The model under review builds one solid part; all positions refer to its coordinate system, in mm. Face numbers are marked on the shaded views. A direction names the side the tool comes from. Coordinates: 2 decimals unless noted, no trailing zeros. Loops run counter-clockwise (first coordinate to the right, second up) from the corner with the lowest first, then second, coordinate; pieces in that order, holes last. Notation, with made-up numbers: M 24.25,59 L 32.25,59 A28 ccw 32.25,80 Z; hole C 16,-11 d6. An arc over 180 degrees is marked long. Return JSON: item names as keys, results as strings.
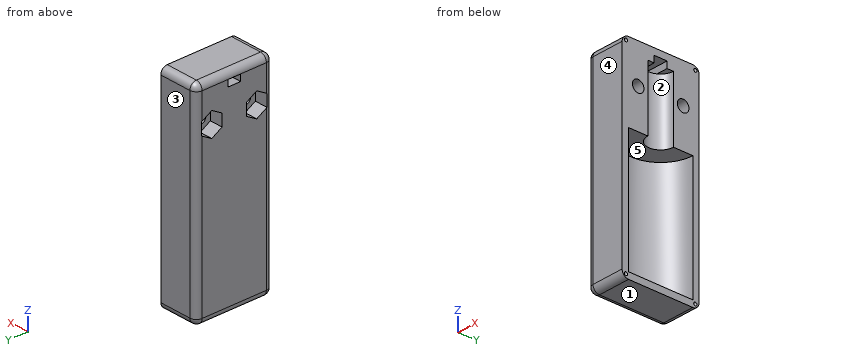
```python
from build123d import *

# Parameters (mm, degrees)
SKETCH1_W               = 6
SKETCH1_H               = 12
BOSS_EXTRUDE1_DEPTH     = 20
SKETCH2_R               = 5
CUT_EXTRUDE1_DEPTH      = 19
SKETCH6_W               = 6
SKETCH6_H               = 12
BOSS_EXTRUDE3_DEPTH     = 12
SKETCH7_R               = 2
CUT_EXTRUDE2_DEPTH      = 10
CUT_EXTRUDE3_DEPTH      = 25.083189158
CUT_EXTRUDE3_DEPTH_BACK = 25.083189158
SKETCH8_W               = 1
SKETCH8_H               = 2
FILLET1_R               = 1
SKETCH10_R              = 0.9
CUT_EXTRUDE4_DEPTH      = 10
CUT_EXTRUDE5_DEPTH      = 2


with BuildPart() as part:
    # Sketch1 → Boss-Extrude1 (new body)
    with BuildSketch(Plane.XY):
        with Locations((3, 6)):
            Rectangle(SKETCH1_W, SKETCH1_H)
    extrude(amount=-BOSS_EXTRUDE1_DEPTH)

    # Sketch2 → Cut-Extrude1 (cut)
    with BuildSketch(Plane.XY):
        with Locations((6, 6)):
            Circle(SKETCH2_R)
    extrude(amount=-CUT_EXTRUDE1_DEPTH, mode=Mode.SUBTRACT)

    # Sketch6 → Boss-Extrude3 (add)
    with BuildSketch(Plane.XY):
        with Locations((3, 6)):
            Rectangle(SKETCH6_W, SKETCH6_H)
    extrude(amount=BOSS_EXTRUDE3_DEPTH)

    # Sketch7 → Cut-Extrude2 (cut)
    with BuildSketch(Plane(origin=(0, 0, 0), x_dir=(-1, 0, 0), z_dir=(0, 0, -1))):
        with Locations((-6, 6)):
            Circle(SKETCH7_R)
    extrude(amount=-CUT_EXTRUDE2_DEPTH, mode=Mode.SUBTRACT)

    # Sketch8 → Cut-Extrude3 (cut, two sides: drawn at the far end of the back side and taken through both)
    with BuildSketch(Plane.ZY.offset(-CUT_EXTRUDE3_DEPTH_BACK)):
        with Locations((10.5, 6)):
            Rectangle(SKETCH8_W, SKETCH8_H)
    extrude(amount=CUT_EXTRUDE3_DEPTH + CUT_EXTRUDE3_DEPTH_BACK, mode=Mode.SUBTRACT)

    # Fillet1
    fillet1_edges = [part.edges().sort_by_distance(p)[0] for p in [
        (3, 0, -20),
        (3, 12, 12),
        (0, 6, 12),
        (3, 0, 12),
        (0, 6, -20),
        (0, 0, -4),
        (0, 12, -4),
        (3, 12, -20),
    ]]
    fillet(fillet1_edges, radius=FILLET1_R - 0.0001)  # a hair under: the kernel refuses the full size

    # Sketch10 → Cut-Extrude4 (cut)
    with BuildSketch(Plane(origin=(6, 0, 0), x_dir=(0, 0, -1), z_dir=(1, 0, 0))):
        with Locations((-6, 9.5)):
            Circle(SKETCH10_R)
    cut_extrude4 = extrude(amount=-CUT_EXTRUDE4_DEPTH, mode=Mode.SUBTRACT)

    # Sketch12 → Cut-Extrude5 (cut)
    with BuildSketch(Plane.ZY):
        Polygon((6.923760431, 7.9), (7.847520861, 9.5), (6.923760431, 11.1), (5.076239569, 11.1), (4.152479139, 9.5), (5.076239569, 7.9), align=None)
    cut_extrude5 = extrude(amount=-CUT_EXTRUDE5_DEPTH, mode=Mode.SUBTRACT)

    # Mirror1: Cut-Extrude4, Cut-Extrude5 across plane
    add(cut_extrude4.mirror(Plane.ZX.offset(6)), mode=Mode.SUBTRACT)
    add(cut_extrude5.mirror(Plane.ZX.offset(6)), mode=Mode.SUBTRACT)

    # Sketch11 → Cut-Revolve1 (revolve, cut)
    with BuildSketch(Plane(origin=(0, 0, -19.4), x_dir=(-1, 0, 0), z_dir=(0, 0, -1))):
        with BuildLine():
            Line((-5.75, 11.4), (-6, 11.4))
            Line((-6, 11.4), (-6, 11.15))
            ThreePointArc((-6, 11.15), (-5.823223305, 11.223223305), (-5.75, 11.4))
        make_face()
    cut_revolve1 = revolve(axis=Axis((5.75, 11.4, -19.4), (1, 0, 0)), mode=Mode.SUBTRACT)

    # Mirror2: Cut-Revolve1 across plane
    add(cut_revolve1.mirror(Plane.ZX.offset(6)), mode=Mode.SUBTRACT)

    # Mirror2 at the second plane: Cut-Revolve1 across plane
    add(cut_revolve1.mirror(Plane.XY.offset(-4)), mode=Mode.SUBTRACT)

    # Mirror2 at the second plane copy 1 sketc → Mirror2 at the second plane copy 1 (revolve, cut)
    with BuildSketch(Plane(origin=(0, 12, 11.4), x_dir=(-1, 0, 0), z_dir=(0, 0, 1))):
        with BuildLine():
            Line((-5.75, 11.4), (-6, 11.4))
            Line((-6, 11.4), (-6, 11.15))
            ThreePointArc((-6, 11.15), (-5.823223305, 11.223223305), (-5.75, 11.4))
        make_face()
    revolve(axis=Axis((5.75, 0.6, 11.4), (1, 0, 0)), mode=Mode.SUBTRACT)


solid = part.part
```
1. Add section B-B on z = 6. Give the boundary of the cut face in (x, y) (3 decimals).
Check values:
{"outline": "M 0,4.1 L 2,4.1 L 2,3.4 L 6,3.4 L 6,4 A2 cw 6,8 L 6,8.6 L 2,8.6 L 2,7.9 L 0,7.9 Z; M 0.005,0.9 A1 ccw 1,0 L 6,0 L 6,1.6 L 2,1.6 L 2,0.9 Z; M 0.005,11.1 L 2,11.1 L 2,10.4 L 6,10.4 L 6,12 L 1,12 A1 ccw Z"}
2. Add section D-D on x = 5. Give the boundary of the cut face in (y, z), plus the area to 3 significant figures.
Check values:
{"outline": "M 0,-19 A1 ccw 1,-20 L 11,-20 A1 ccw 12,-19 L 12,11 A1 ccw 11,12 L 1,12 A1 ccw 0,11 Z; hole M 1.1,-19 L 10.9,-19 L 10.9,0 L 7.73,0 L 7.73,10 L 7,10 L 7,11 L 5,11 L 5,10 L 4.27,10 L 4.27,0 L 1.1,0 Z; hole C 2.5,6 d1.8; hole C 9.5,6 d1.8", "area": "155 mm²"}
3. The part is to be moulded in two halves that separate along Z. For the marked faces 1, 2 and 3, say which applies: released by +Z, released by -Z, zero draft, split by the parting line, or undercut.
Check values:
{"face 1": "released by -Z", "face 2": "undercut", "face 3": "zero draft"}
4. To check wall thickness, follow line 1 (Y direction, x = 3.45, z = 6); line 2 (Z direction, x = 3.15, y = 2.5); line 3 (Z direction, x = 2.25, y = 9). State the ranges of each line that lie inside material, in increasing order.
Check values:
{"line 1": "0 to 1.6, 3.4 to 8.6, 10.4 to 12", "line 2": "-20 to -19, 0 to 5.1, 6.9 to 12", "line 3": "-20 to -19, 0 to 5.25, 6.75 to 12"}
5. Machinability: for the marked faces 4 and 5, which of the approach directions +Z, -Z, +X, -X, +Y, -Y give a long, thin tool a straight path to every point of the face, cutting with its end or side? Answer none if there is none.
Check values:
{"face 4": "+Z, -Z, +X, -X, -Y", "face 5": "+X"}
6. Add section C-C on x = 3.5. Give the boundary of the cut face in (y, z).
Check values:
{"outline": "M 0,-19 A1 ccw 1,-20 L 11,-20 A1 ccw 12,-19 L 12,11 A1 ccw 11,12 L 1,12 A1 ccw 0,11 Z; hole C 2.5,6 d1.8; hole M 1.67,-19 L 10.33,-19 L 10.33,0 L 1.67,0 Z; hole M 5,10 L 7,10 L 7,11 L 5,11 Z; hole C 9.5,6 d1.8"}
7. Insertion check: pin 1 Ø3.5 at (y, z) = (3, 5.5) entering from -X; pin 2 Ø3 at (y, z) = (9, -14) entering from +X; pin 3 Ø1 at (y, z) = (8.5, 5.5) entering from -X. Each pin has a flat end and moves straight along its axis. Give the tip position at first contact, or say it passes through.
Check values:
{"pin 1": "x = 0", "pin 2": "x = 3.82", "pin 3": "x = 2"}
